Source: CAD feature listing. Evaluate the final solid. Frame: model axes, mm. Round coordinates to 2 decimals unless told otherwise and drop trailing zeros. Write each loop counter-clockwise with the first axis right and the second up, starting at its lowest first coordinate (ties: lowest second). Pieces come first, ordered by that corner, then holes. Notation, with made-up numbers: (11, 88.25) - (19, 88.25) arc R35 cw to (19, 126.25) - close; hole circle Ø4 at (37.5, 10.5). An arc over 180 degrees is marked (long way). Write item = value, one per line. Start each with the question number.
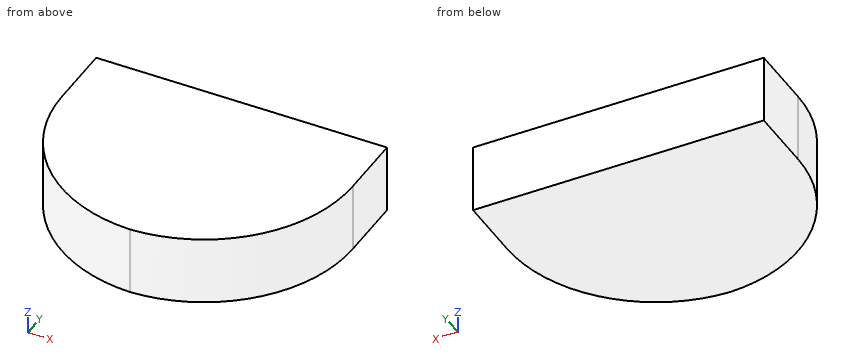
```python
from build123d import *

# Parameters (mm, degrees)
F0_W        = 76
F0_H        = 56
F1_DEPTH    = 18
F2_T1_DEPTH = 212.344191771


# Not quite as in the source:
# - a fillet or chamfer that OpenCascade refuses, or shapes differently, is made with other operations: its cross-section is extruded or revolved along the edge and cut away or added


with BuildPart() as f1:
    # F0 (on Top) → F1 (new body)
    with BuildSketch(Plane.XY):
        with Locations((2.4067710042, -5.2896709442)):
            Rectangle(F0_W, F0_H)
    extrude(amount=F1_DEPTH)

    # F2: fillet of radius 38.8688383542 on 2 edges, made by hand

    # F2_s2 → F2_t1 (cut)
    with BuildSketch(Plane.XY.offset(-97.1720958855)):
        with BuildLine():
            ThreePointArc((-35.5932289958, 5.57916741), (-24.2088098187, -21.9052517671), (3.2756093584, -33.2896709442))
            Line((3.2756093584, -33.2896709442), (-35.5932289958, -33.2896709442))
            Line((-35.5932289958, -33.2896709442), (-35.5932289958, 5.57916741))
        make_face()
        with BuildLine():
            ThreePointArc((40.4067710042, 5.57916741), (29.0223518271, -21.9052517671), (1.53793265, -33.2896709442))
            Line((1.53793265, -33.2896709442), (40.4067710042, -33.2896709442))
            Line((40.4067710042, -33.2896709442), (40.4067710042, 5.57916741))
        make_face()
    extrude(amount=F2_T1_DEPTH, mode=Mode.SUBTRACT)


solid = f1.part
```
(1) Ray query, L1, parallel to X at y = -26.5, z = 8; L2, parallel to Y at x = -31.5, z = 16.5; L3, parallel to Y at x = 20.5, z = 14. Return the intervals inside material, ascending. Write a range as from..to.
(2) Section B-B (y = -20). Return the cut outline in (x, z).
(3) Section A-A (z = 13). Return the cut outline in (x, y), plus the area to 3 significant figures.
(4) Section C-C (x = -16). Return the cut outline in (y, z).
(5) Contact query for flat-ended pins moving along their axis: P1, Ø1, axis at x = -12, y = -4, coming from the -Z side; P2, Ø5, axis at x = -7.5, z = 9.5, coming from the -Y side; P3, Ø1.5, axis at x = -2, z = 11.5, coming from the -Y side; P4, Ø1, axis at y = -25.5, z = 13.5, coming from the +X side. Output: stop coordinate, or through.
Solution:
q1.L1 = -18.67..23.49
q1.L2 = -11.78..22.71
q1.L3 = -28.35..22.71
q2.outline = (-25.99, 0) - (30.8, 0) - (30.8, 18) - (-25.99, 18) - close
q3.outline = (-35.59, 5.58) arc R38.87 ccw to (2.41, -33.28) arc R38.87 ccw to (40.41, 5.58) - (40.41, 22.71) - (-35.59, 22.71) - close
q3.area = 3,610 mm^2
q4.outline = (-28.17, 0) - (22.71, 0) - (22.71, 18) - (-28.17, 18) - close
q5.P1 = 0
q5.P2 = -32.4
q5.P3 = -33.03
q5.P4 = 25.53
